```python
from build123d import *

# Parameters (mm, degrees)
F0_W     = 254
F0_H     = 50.8
F1_DEPTH = 25.4
F3_W     = 76.2
F3_H     = 76.2


with BuildPart() as f1:
    # F0 (on Front) → F1 (new body, symmetric)
    with BuildSketch(Plane.XZ):
        with Locations((127, 25.4)):
            Rectangle(F0_W, F0_H)
    extrude(amount=F1_DEPTH, both=True)

    # F3 (on Front) → F4 (revolve)
    with BuildSketch(Plane.XZ):
        with Locations((-38.1, 38.1)):
            Rectangle(F3_W, F3_H)
    revolve(axis=Axis((0, 0, 56.434907), (0, 0, 1)))


solid = f1.part
```
Can you work these out from the model? Positions are in its coordinate system, mm. A direction names the side the tool comes from. Round coordinates to 2 decimals unless told otherwise and drop trailing zeros. Loops run counter-clockwise (first coordinate to the right, second up) from the corner with the lowest first, then second, coordinate; pieces in that order, holes last. Notation, with made-up numbers: (-16.75, 14) -> (-4.75, 14) arc R18 cw to (-4.75, 34) -> close; hole circle Ø3 at (66, 24.25). An arc over 180 degrees is marked (long way). One line per item, written item: value. Start each with the question number.
1. If we section it at C-C, the plane x = 191: Write out the boundary of the cut face in (y, z).
2. If we section it at A-A, the plane y = 0: Write out the boundary of the cut face in (x, z), then the cut area to 3 significant figures.
3. For pin 1 (3 mm diameter, centred on y = -14.5, z = 57, fed in from +X); pin 2 (10 mm diameter, centred on x = -14.5, z = 60, fed in from +Y); pin 3 (6 mm diameter, centred on x = -29.5, z = 55, fed in from +Y), each with a flat end and sliding along its axis, tell me the tip position at first contact or that it passes through.
4. If we section it at D-D, the plane z = 16: Write out the boundary of the cut face in (x, y), then the cut area to 3 significant figures.
5. For faces 1 (the flat face through (55, -1, 0)), 2 (the flat face through (162, 25.4, 26)), 3 (the flat face through (162, -25.4, 26)), which set-ups out of +Z, -Z, +X, -X, +Y, -Y let a thin tool reach every point of the face, with its end or its side?
6. If we section it at B-B, the plane z = 70: Write out the boundary of the cut face in (x, y), then the cut area to 3 significant figures.
7. If I drill on probe 1 along Y at (x, z) = (86, 18); probe 2 along X at (y, z) = (2, 19); probe 3 along Z at (x, y) = (196, 3.5), over which ranges is the centre line in solid material (lowest first)?
Calculated:
1. outline: (-25.4, 0) -> (25.4, 0) -> (25.4, 50.8) -> (-25.4, 50.8) -> close
2. outline: (-76.2, 0) -> (254, 0) -> (254, 50.8) -> (76.2, 50.8) -> (76.2, 76.2) -> (-76.2, 76.2) -> close
2. area: 20,600 mm²
3. pin 1: stops at x = 75.08
3. pin 2: stops at y = 75.61
3. pin 3: stops at y = 71.44
4. outline: (71.84, -25.4) -> (254, -25.4) -> (254, 25.4) -> (71.84, 25.4) arc R76.2 ccw (long way) to start
4. area: 27,300 mm²
5. face 1: -Z, +X, -X, +Y, -Y
5. face 2: +Z, -Z, +X, +Y
5. face 3: +Z, -Z, +X, -Y
6. outline: circle Ø152.4 at (0, 0)
6. area: 18,200 mm²
7. probe 1: y = -25.4 to 25.4
7. probe 2: x = -76.17 to 254
7. probe 3: z = 0 to 50.8
